Work out the finished part from the listing and answer in its coordinate system (mm). Face numbers are marked on the shaded views. A direction names the side the tool comes from. Give positions to 0.01 mm unless a question says otherwise; leave off trailing zeros. Write each loop counter-clockwise with the first axis right and the second up, starting at its lowest first coordinate (ties: lowest second). Pieces come first, ordered by that corner, then holes. Notation, with made-up numbers: (-28, -38) -> (22, -38) arc R37 cw to (22, 0) -> close; hole circle Ø9 at (1.5, 42.5). An arc over 180 degrees is marked (long way). Use a Markdown table: item, result. Add a question column.
Q1. Section C-C, the plane x = 23 is taken. Give the vertices of the cut face in (y, z), plus the area to 3 significant figures.
Q2. For the marked faces 1 and 2, determine the directions among +Z, -Z, +X, -X, +Y, -Y from which every point of the face is accessible in a straight line to the end or side of a thin tool.
Q3. Section D-D, the plane y = 15 is taken. Give the vertices of the cut face in (x, z).
Q4. Consider line 1 (Y direction, x = 0, z = 2.5); line 2 (Y direction, x = 0, z = 6.25); line 3 (Y direction, x = -23, z = 11.8). Determine where each line is inside the solid, lowest interval first.
Q5. Section A-A, the plane y = 0 is taken. Give the vertices of the cut face in (x, z).
Q6. Each of these flat-tipped pins is pushed along its axis until it touches: pin 1 Ø1.9 at (x, y) = (5.66, -5.66) entering from +Z; pin 2 Ø1.8 at (x, y) = (8, 1) entering from +Z; pin 3 Ø5 at (x, y) = (23.5, 14.5) entering from -Z; pin 4 Ø4 at (y, z) = (-19, 7) entering from +X. Where does it stop, or does it pass through?
Autodesk Inventor part; units mm, degrees
ref_plane "YZ Plane" through (0, 0, 0) normal (1, 0, 0) x (0, 1, 0)
ref_plane "XZ Plane" through (0, 0, 0) normal (0, 1, 0) x (-1, 0, 0)
ref_plane "XY Plane" through (0, 0, 0) normal (0, 0, 1) x (1, 0, 0)
sketch "Эскиз1" plane through (0, 0, 0) normal (0, 0, 1) x (1, 0, 0)
  circle A0 centre (0, 0) radius 3.75
  circle A1 centre (0, 0) radius 10.8
  circle A2 centre (0, 0) radius 2.85
  circle A3 centre (-5.6569, 5.6569) radius 1.2
  circle A4 centre (-8, 0) radius 1.2
  circle A5 centre (-5.6569, -5.6569) radius 1.2
  circle A6 centre (0, -8) radius 1.2
  circle A7 centre (5.6569, -5.6569) radius 1.2
  circle A8 centre (8, 0) radius 1.2
  circle A9 centre (5.6569, 5.6569) radius 1.2
  circle A10 centre (0, 8) radius 1.2
  circle A11 centre (0, 0) radius 11
extrude "Выдавливание1" add sketch "Эскиз1" along normal blind 3 contours A1 | A11
sketch "Эскиз6" plane through (0, 0, 3) normal (0, 0, 1) x (1, 0, 0)
  circle A0 centre (0, 0) radius 3.75
  circle A1 centre (0, 0) radius 35
  circle A2 centre (0, 0) radius 11
  circle A3 centre (0, 0) radius 3.75
  circle A4 centre (-5.6569, 5.6569) radius 1.2
  circle A5 centre (-8, 0) radius 1.2
  circle A6 centre (-5.6569, -5.6569) radius 1.2
  circle A7 centre (0, -8) radius 1.2
  circle A8 centre (5.6569, -5.6569) radius 1.2
  circle A9 centre (8, 0) radius 1.2
  circle A10 centre (5.6569, 5.6569) radius 1.2
  circle A11 centre (0, 8) radius 1.2
  dimension "d21" = 70
extrude "Выдавливание6" add sketch "Эскиз6" along normal blind 10 contours A1 | A2
sketch "Эскиз7" plane through (0, 0, 13) normal (0, 0, 1) x (1, 0, 0)
  circle A0 centre (0, 8) radius 1.2
  circle A1 centre (0, 8) radius 3
  point P0 (0, 0)
  dimension "d24" = 6
extrude "Выдавливание7" cut sketch "Эскиз7" against normal blind 5 contours A0 | A1
pattern_circular "Круговой массив2" count 8 over 360 about axis through (0, 0, 0) along (0, 0, 1) of "Выдавливание7"
sketch "Эскиз8" plane through (0, 0, 13) normal (0, 0, 1) x (1, 0, 0)
  line L0 (0, 0) -> (-23, 0) construction
  line L1 (-23, 0) -> (-23, 15) construction
  circle A0 centre (-23, 15) radius 2
  dimension "d30" = 23
  dimension "d31" = 15
  dimension "d32" = 4
extrude "Выдавливание8" cut sketch "Эскиз8" against normal through all
sketch "Эскиз9" plane through (0, 0, 3) normal (0, 0, -1) x (-1, 0, 0)
  circle A0 centre (23, 15) radius 2
  circle A1 centre (23, 15) radius 3
  point P0 (0, 0)
  dimension "d35" = 6
extrude "Выдавливание9" cut sketch "Эскиз9" against normal blind 5 contours A0 | A1
mirror "Зеркальное отражение3" about plane through (0, 0, 0) normal (0, 1, 0) of "Выдавливание9", "Выдавливание8"
mirror "Зеркальное отражение4" about plane through (0, 0, 0) normal (1, 0, 0) of "Выдавливание9", "Зеркальное отражение3", "Выдавливание8"
properties part number "000.005.004.003 - ПОВОРОТНЫЙ ДИСК" material "Пластик АБС"
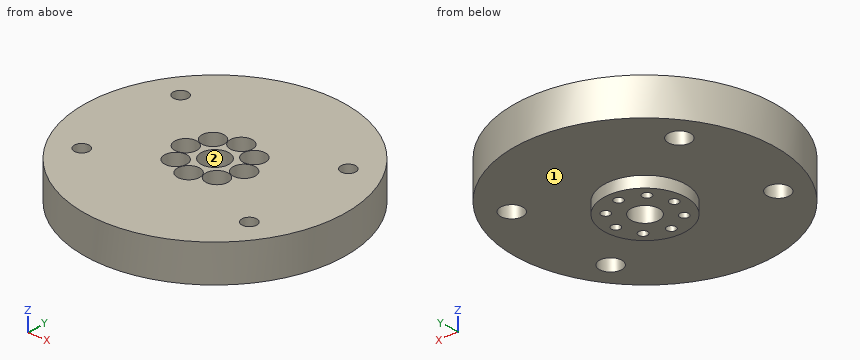
Result set:
| question | item | result |
|---|---|---|
| 1 | outline | (-26.38, 3) -> (-18, 3) -> (-18, 8) -> (-17, 8) -> (-17, 13) -> (-26.38, 13) -> close; (-13, 8) -> (-12, 8) -> (-12, 3) -> (12, 3) -> (12, 8) -> (13, 8) -> (13, 13) -> (-13, 13) -> close; (17, 8) -> (18, 8) -> (18, 3) -> (26.38, 3) -> (26.38, 13) -> (17, 13) -> close |
| 1 | area | 428 mm2 |
| 2 | face 1 | -Z |
| 2 | face 2 | +Z, -Z |
| 3 | outline | (-31.62, 3) -> (-26, 3) -> (-26, 8) -> (-25, 8) -> (-25, 13) -> (-31.62, 13) -> close; (-21, 8) -> (-20, 8) -> (-20, 3) -> (20, 3) -> (20, 8) -> (21, 8) -> (21, 13) -> (-21, 13) -> close; (25, 8) -> (26, 8) -> (26, 3) -> (31.62, 3) -> (31.62, 13) -> (25, 13) -> close |
| 4 | line 1 | y = -11 to -9.2, -6.8 to -3.75, 3.75 to 6.8, 9.2 to 11 |
| 4 | line 2 | y = -35 to -9.2, -6.8 to -3.75, 3.75 to 6.8, 9.2 to 35 |
| 4 | line 3 | y = -26.38 to -17, -13 to 13, 17 to 26.38 |
| 5 | outline | (-35, 3) -> (-11, 3) -> (-11, 0) -> (-9.2, 0) -> (-9.2, 8) -> (-11, 8) -> (-11, 13) -> (-35, 13) -> close; (-6.8, 0) -> (-3.75, 0) -> (-3.75, 13) -> (-5, 13) -> (-5, 8) -> (-6.8, 8) -> close; (3.75, 0) -> (6.8, 0) -> (6.8, 8) -> (5, 8) -> (5, 13) -> (3.75, 13) -> close; (9.2, 0) -> (11, 0) -> (11, 3) -> (35, 3) -> (35, 13) -> (11, 13) -> (11, 8) -> (9.2, 8) -> close |
| 6 | pin 1 | passes through |
| 6 | pin 2 | stops at z = 8 |
| 6 | pin 3 | stops at z = 3 |
| 6 | pin 4 | stops at x = 30.59 |
